Source: CAD feature listing. Evaluate the final solid. Frame: model axes, mm. Face numbers are marked on the shaded views. A direction names the side the tool comes from. Give positions to 0.01 mm unless a question says otherwise; leave off trailing zeros. Write each loop counter-clockwise with the first axis right and the second up, starting at its lowest first coordinate (ties: lowest second). Pieces come first, ordered by that corner, then holes. Notation, with made-up numbers: (-4.5, 42) -> (27.5, 42) arc R21 cw to (27.5, 46) -> close; hole circle Ø3 at (56, 20). An arc over 180 degrees is marked (long way). Use one line per item in the form item = value. Start each with the question number.
(1) First-contact query: P1, Ø8, axis at y = -87.5, z = 3.5, coming from the -X side; P2, Ø22, axis at x = 0.5, y = 126, coming from the -Z side; P3, Ø6, axis at y = 71.5, z = 40, coming from the +X side. Flat tips, straight axial feed; report the tip coordinate or a pass-through.
(2) Draft query along Y for the marked faces 4, 5 and 6. Return one class per face: pulls with the +Y half, pulls with the -Y half, needs draft (parallel to the pull), parting line crosses it, or undercut.
(3) Cut plane B-B, the plane x = 165.5. Output: boundary loops of the cut face in (y, z), and give its area (3 significant figures).
(4) Cut plane A-A, the plane z = 74. Output: boundary loops of the cut face in (x, y), and give its area (3 significant figures).
(5) Material intervals for line 1 along Y through (x, z) = (182.5, 38); line 2 along Y through (x, z) = (-177, 87); line 3 along X through (y, z) = (-199, 26.5), sorted ascending. Write a range as from..to.
(6) Cut plane C-C, the plane y = -124. Output: boundary loops of the cut face in (x, z).
(7) Set-up query: the marked faces 1, 2 and 3. Return all of +Z, -Z, +X, -X, +Y, -Y with unobstructed straight access to the full face (end or side cutting, diameter ignored); none if empty.
Autodesk Inventor part; units mm, degrees
ref_plane "Work Plane1" through (0, -300, 0) normal (1, 0, 0) x (0, 0, -1)
ref_plane "YZ Plane" through (0, 0, 0) normal (1, 0, 0) x (0, 1, 0)
ref_plane "XZ Plane" through (0, 0, 0) normal (0, 1, 0) x (-1, 0, 0)
sketch "Sketch1" plane through (0, 0, 0) normal (0, 0, 1) x (1, 0, 0)
  line L0 (150, 300) -> (-150, 300)
  line L1 (-150, 300) -> (-150, -300)
  line L2 (-150, -300) -> (150, -300)
  line L3 (150, -300) -> (150, 300)
  line L4 (150, 300) -> (-150, -300) construction
  line L5 (-150, 300) -> (150, -300) construction
  point P0 (0, 0)
  dimension "d0" = 300
  dimension "d1" = 600
extrude "Extrusion1" add sketch "Sketch1" along normal blind 100
sketch "Sketch2" plane through (0, 0, 100) normal (0, 0, 1) x (1, 0, 0)
  line L0 (-150, 300) -> (-150, -300)
  line L1 (-150, -300) -> (-230, -300)
  line L2 (-230, -300) -> (-230, -260)
  line L3 (-230, -260) -> (-150, -260)
  line L4 (-150, -260) -> (-150, -300)
  point P0 (0, 0)
  dimension "d4" = 80
  dimension "d5" = 40
extrude "Extrusion2" add sketch "Sketch2" against normal up to surface (100 mm away)
sketch "Sketch3" plane through (0, 0, 100) normal (0, 0, 1) x (1, 0, 0)
  line L0 (-150, 300) -> (-150, -260)
  line L1 (-150, -260) -> (-150, -300) construction
  line L2 (150, -300) -> (-230, -300)
  line L3 (-150, -260) -> (-230, -260)
  line L4 (-230, -260) -> (-150, -300) construction
  line L5 (-150, -260) -> (-230, -300) construction
  line L6 (-182.2361, -289.15) -> (-197.7639, -289.15)
  line L7 (-197.7639, -289.15) -> (-197.7639, -270.85) construction
  line L8 (-197.7639, -270.85) -> (-182.2361, -270.85)
  line L9 (-182.2361, -289.15) -> (-197.7639, -270.85) construction
  line L10 (-197.7639, -289.15) -> (-182.2361, -270.85) construction
  arc A0 (-197.7639, -270.85) -> (-197.7639, -289.15) centre (-190, -280) ccw
  arc A1 (-182.2361, -289.15) -> (-182.2361, -270.85) centre (-190, -280) ccw
  point P0 (0, 0)
  dimension "d9" = 18.3
extrude "Extrusion3" cut sketch "Sketch3" against normal up to surface (100 mm away)
ref_plane "Work Plane1" through (0, -300, 0) normal (1, 0, 0) x (0, 0, -1)
mirror "Mirror1" about plane through (0, -300, 0) normal (1, 0, 0) of "Extrusion2", "Extrusion3"
ref_plane "Work Plane2" through (-150, 0, 0) normal (0, 1, 0) x (1, 0, 0)
mirror "Mirror2" about plane through (-150, 0, 0) normal (0, 1, 0) of "Extrusion2", "Extrusion3", "Mirror1"
sketch "Sketch4" plane through (-230, 300, 0) normal (0, 1, 0) x (1, 0, 0)
  line L0 (240, 7.5) -> (220, 7.5)
  line L1 (220, 7.5) -> (220, -7.5)
  line L2 (220, -7.5) -> (240, -7.5)
  line L3 (240, -7.5) -> (240, 7.5)
  line L4 (240, 7.5) -> (220, -7.5) construction
  line L5 (220, 7.5) -> (240, -7.5) construction
  point P0 (230, 0)
  dimension "d12" = 20
  dimension "d13" = 15
extrude "Extrusion4" cut sketch "Sketch4" against normal through all
properties part number "backplate"
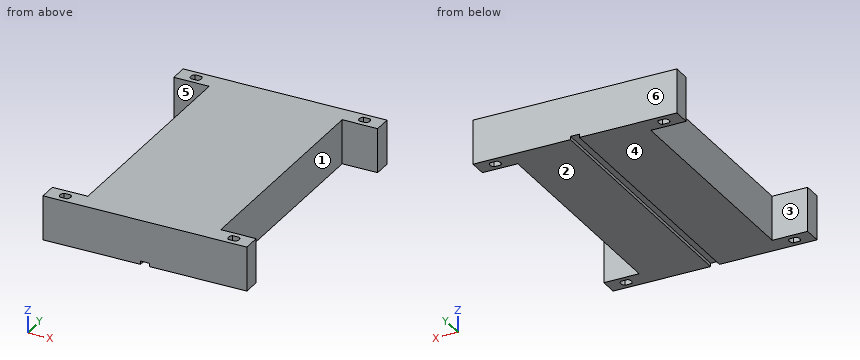
Geometry says:
q1.P1 = -150
q1.P2 = 0
q1.P3 = 150
q2.face_4 = needs draft
q2.face_5 = undercut
q2.face_6 = pulls with the +Y half
q3.outline = (-300, 0) -> (-260, 0) -> (-260, 100) -> (-300, 100) -> close; (260, 0) -> (300, 0) -> (300, 100) -> (260, 100) -> close
q3.area = 8,000 mm^2
q4.outline = (-230, -300) -> (230, -300) -> (230, -260) -> (150, -260) -> (150, 260) -> (230, 260) -> (230, 300) -> (-230, 300) -> (-230, 260) -> (-150, 260) -> (-150, -260) -> (-230, -260) -> close; hole (-197.76, -289.15) -> (-182.24, -289.15) arc R12 ccw to (-182.24, -270.85) -> (-197.76, -270.85) arc R12 ccw to start; hole (-197.76, 270.85) -> (-182.24, 270.85) arc R12 ccw to (-182.24, 289.15) -> (-197.76, 289.15) arc R12 ccw to start; hole (182.24, -289.15) -> (197.76, -289.15) arc R12 ccw to (197.76, -270.85) -> (182.24, -270.85) arc R12 ccw to start; hole (182.24, 270.85) -> (197.76, 270.85) arc R12 ccw to (197.76, 289.15) -> (182.24, 289.15) arc R12 ccw to start
q4.area = 191,000 mm^2
q5.line_1 = -300..-289.15, -270.85..-260, 260..270.85, 289.15..300
q5.line_2 = -300..-260, 260..300
q5.line_3 = -150..150
q6.outline = (-150, 0) -> (-10, 0) -> (-10, 7.5) -> (10, 7.5) -> (10, 0) -> (150, 0) -> (150, 100) -> (-150, 100) -> close
q7.face_1 = +Z, -Z, +X
q7.face_2 = -Z, +X, -X, +Y, -Y
q7.face_3 = +Z, -Z, -X
